Could you check a few things on this model? Use its own coordinates, in mm. A direction names the side the tool comes from. Coordinates: 2 decimals unless noted, no trailing zeros. Order: outer loops, then holes, each group sorted by start corner. A loop starts at its lowest first (then second) coordinate and runs counter-clockwise, first axis right, second up. Notation, with made-up numbers: (-25, 86) - (15, 86) arc R27 ccw to (15, 120) - close; hole circle Ø10 at (-12, -13). An arc over 180 degrees is marked (long way). Answer as CSV lines item,"result". Start each with the question number.
1. I want a section at B-B, the plane z = -39. List the corners of the cut face in (x, y) for me.
2. For pin 1 (1 mm diameter, centred on y = 2.5, z = 9.5, fed in from +X); pin 2 (5.5 mm diameter, centred on x = 22, y = 1.5, fed in from -Z); pin 3 (4 mm diameter, centred on y = -3.5, z = -13.5, fed in from +X), each with a flat end and sliding along its axis, tell me the tip position at first contact or that it passes through.
3. I need wall thicknesses on probe 1 along Z at (x, y) = (-4.5, 4.25); probe 2 along Y at (x, z) = (0, -1); probe 3 along X at (y, z) = (-2.75, -43.5). Which ranges of each line are inside material? Lowest first, please.
4. I want a section at A-A, the plane y = 0. List the corners of the cut face in (x, z) for me.
5. I want a section at C-C, the plane x = 18.5. List the corners of the cut face in (y, z) for me, and give its area (3 significant figures).
6. I want a section at D-D, the plane z = 14. List the corners of the cut face in (x, y) for me.
7. For faces 1 (the face through (30, -9.15, 10)), 2 (the face through (-0.683, 3.075, -26.721)), which set-ups out of +Z, -Z, +X, -X, +Y, -Y let a thin tool reach every point of the face, with its end or its side?
from build123d import *

# Parameters (mm, degrees)
SALIENTE_EXTRUIR1_DEPTH = 20
SALIENTE_EXTRUIR2_DEPTH = 20
CROQUIS3_R              = 3.15
SALIENTE_EXTRUIR3_DEPTH = 55.4
CHAFL_N1_SIZE           = 1.2
CHAFL_N1_SIZE2          = 0.692820323


with BuildPart() as part:
    # Croquis1 → Saliente-Extruir1 (new body)
    with BuildSketch(Plane.XY):
        with BuildLine():
            Line((0.57794053, 7.728420585), (63.919718915, 2.991646678))
            ThreePointArc((63.919718915, 2.991646678), (66.696, 0), (63.919718915, -2.991646678))
            Line((63.919718915, -2.991646678), (0.57794053, -7.728420585))
            ThreePointArc((0.57794053, -7.728420585), (-7.75, 0), (0.57794053, 7.728420585))
        make_face()
    extrude(amount=SALIENTE_EXTRUIR1_DEPTH)

    # Croquis2 → Saliente-Extruir2 (add)
    with BuildSketch(Plane.XY):
        with BuildLine():
            Line((0, 9.15), (58.946, 9.15))
            ThreePointArc((58.946, 9.15), (68.096, 0), (58.946, -9.15))
            Line((58.946, -9.15), (0, -9.15))
            ThreePointArc((0, -9.15), (-9.15, 0), (0, 9.15))
        make_face()
    extrude(amount=SALIENTE_EXTRUIR2_DEPTH)

    # Croquis3 → Saliente-Extruir3 (add)
    with BuildSketch(Plane(origin=(0, 0, 0), x_dir=(-1, 0, 0), z_dir=(0, 0, -1))):
        with Locations(Location((0, 0, 0), (0, 0, 180))):
            Circle(CROQUIS3_R)
    extrude(amount=SALIENTE_EXTRUIR3_DEPTH)

    # Chafl_n1
    chafl_n1_edges = [part.edges().sort_by_distance(p)[0] for p in [
        (-3.15, 0, -55.4),
    ]]
    chafl_n1_side = [part.faces().sort_by_distance(p)[0] for p in [
        (-3.15, 0, -27.7),
    ]]
    chamfer(chafl_n1_edges, length=CHAFL_N1_SIZE, length2=CHAFL_N1_SIZE2, reference=chafl_n1_side[0])


solid = part.part
Solved:
1,outline,"circle Ø6.3 at (0, 0)"
2,pin 1,"stops at x = 67.87"
2,pin 2,"stops at z = 0"
2,pin 3,"stops at x = 2.77"
3,probe 1,"z = 0 to 20"
3,probe 2,"y = -3.15 to 3.15"
3,probe 3,"x = -1.54 to 1.54"
4,outline,"(-9.15, 0) - (-3.15, 0) - (-3.15, -54.2) - (-2.46, -55.4) - (2.46, -55.4) - (3.15, -54.2) - (3.15, 0) - (68.1, 0) - (68.1, 20) - (-9.15, 20) - close"
5,outline,"(-9.15, 0) - (9.15, 0) - (9.15, 20) - (-9.15, 20) - close"
5,area,"366 mm2"
6,outline,"(0, -9.15) - (58.95, -9.15) arc R9.15 ccw to (58.95, 9.15) - (0, 9.15) arc R9.15 ccw to start"
7,face 1,"+Z, -Z, +X, -X, -Y"
7,face 2,"-Z"
